Geometry check sheet. Reference: the model listing, model coordinates, mm. Face numbers are marked on the shaded views. A direction names the side the tool comes from. Round coordinates to 2 decimals unless told otherwise and drop trailing zeros. Write each loop counter-clockwise with the first axis right and the second up, starting at its lowest first coordinate (ties: lowest second). Pieces come first, ordered by that corner, then holes. Notation, with made-up numbers: M 48.5,72.5 L 74.5,72.5 A16 cw 74.5,101.5 Z; hole C 28,62 d6. An arc over 180 degrees is marked long. One line per item, written item: value. Start each with the question number.
1. Section check B-B (y = 34.5). Record the boundary of the cut face in (x, z).
2. Section check A-A (y = 82.5). Record the boundary of the cut face in (x, z), and give its area (3 significant figures).
3. Scan lines: probe 1 along X at (y, z) = (14.5, -3.25); probe 2 along X at (y, z) = (-78, 1); probe 3 along Y at (x, z) = (-19, -2.75). Record each from-to range of solid material in increasing order. Write a range as [from, to].
4. Release check for a two-part mould opening along Y. For the marked faces 5, 6 and 7 record: pulls with the +Y half, pulls with the -Y half, needs draft (parallel to the pull), parting line crosses it, or undercut.
5. Access from +Z, -Z, +X, -X, +Y, -Y to the whole of each face (thin tool, end or side, straight path). Record for the marked faces 1, 2, 3 and 4.
6. Depth check by flat-ended pin: P1, Ø6, axis at y = -48.5, z = -2, coming from the +X side; P2, Ø5, axis at y = -47.5, z = -4, coming from the -X side; P3, Ø5, axis at y = 56.5, z = 0.5, coming from the -X side. Enter the tip coordinate at first touch or a pass-through.
from build123d import *

# Parameters (mm, degrees)
SKETCH_1_W          = 49.8
SKETCH_1_H          = 190
EXTRUDE_1_DEPTH     = 5
CUT_EXTRUDE_1_DEPTH = 99.71681721
FILLET_1_R          = 5
CUT_EXTRUDE_2_DEPTH = 99.71681721
CHAMFER_2_SIZE      = 20
CUT_EXTRUDE_6_REACH = 100.717
SKETCH_7_R          = 2.1
SKETCH_3_W          = 30.2
SKETCH_3_H          = 6.2
CUT_EXTRUDE_7_DEPTH = 49
CHAMFER_3_SIZE      = 5
SKETCH_9_R          = 3.7
CUT_EXTRUDE_8_DEPTH = 5


with BuildPart() as part:
    # 草图1 → 凸台-拉伸1 (new, symmetric)
    with BuildSketch(Plane.XY):
        Rectangle(SKETCH_1_W, SKETCH_1_H)
    extrude(amount=EXTRUDE_1_DEPTH, both=True)

    # 草图4 → 切除-拉伸1 (cut, through all)
    with BuildSketch(Plane(origin=(0, 0, -5), x_dir=(-1, 0, 0), z_dir=(0, 0, -1))):
        Polygon((-24.9, 62.5), (-15, 45.352697005), (-15, -45.352697005), (-24.9, -62.5), align=None)
        Polygon((24.9, -62.5), (24.9, 62.5), (15, 45.352697005), (15, -45.352697005), align=None)
    extrude(amount=-CUT_EXTRUDE_1_DEPTH, mode=Mode.SUBTRACT)

    # 圆角1
    fillet_1_edges = [part.edges().sort_by_distance(p)[0] for p in [
        (24.9, -62.5, 0),
        (24.9, 62.5, 0),
        (15, 45.352697005, 0),
        (15, -45.352697005, 0),
        (-24.9, -62.5, 0),
        (-15, -45.352697005, 0),
        (-15, 45.352697005, 0),
        (-24.9, 62.5, 0),
        (24.9, -95, 0),
        (-24.9, -95, 0),
        (-24.9, 95, 0),
        (24.9, 95, 0),
    ]]
    fillet(fillet_1_edges, radius=FILLET_1_R)

    # 草图5 → 切除-拉伸2 (cut, through all)
    with BuildSketch(Plane(origin=(0, 0, -5), x_dir=(-1, 0, 0), z_dir=(0, 0, -1))):
        Polygon((-19.9, 90), (-19.9, 63.839745962), (-10, 46.692442967), (-10, 2.5), (-5, 2.5), (-5, 90), align=None)
        Polygon((5, 90), (19.9, 90), (19.9, 63.839745962), (10, 46.692442967), (10, 2.5), (5, 2.5), align=None)
        Polygon((19.9, -90), (19.9, -63.839745962), (10, -46.692442967), (10, -2.5), (5, -2.5), (5, -90), align=None)
        Polygon((-5, -90), (-19.9, -90), (-19.9, -63.839745962), (-10, -46.692442967), (-10, -2.5), (-5, -2.5), align=None)
    extrude(amount=-CUT_EXTRUDE_2_DEPTH, mode=Mode.SUBTRACT)

    # 倒角2
    # the kernel refuses this chamfer: 20 mm, written as the material it adds along each edge
    with BuildSketch(Plane(origin=(-19.9, 90, -5), x_dir=(-0.027495876610586147, -0.9996219169112968, 0), z_dir=(0, 0, 1))) as chamfer_2_piece_1:
        Polygon((CHAMFER_2_SIZE * 0.999621916911, CHAMFER_2_SIZE * 0.0274958766106), (-CHAMFER_2_SIZE * 0.0274958766106, CHAMFER_2_SIZE * 0.999621916911), (0, 0), align=None)
    extrude(amount=10)
    with BuildSketch(Plane(origin=(19.9, 90, -5), x_dir=(0.027495876610586147, -0.9996219169112968, 0), z_dir=(0, 0, 1))) as chamfer_2_piece_2:
        Polygon((CHAMFER_2_SIZE * 0.999621916911, -CHAMFER_2_SIZE * 0.0274958766106), (-CHAMFER_2_SIZE * 0.0274958766106, -CHAMFER_2_SIZE * 0.999621916911), (0, 0), align=None)
    extrude(amount=10)

    # 草图7 → 切除-拉伸6 (cut, up to next)
    with BuildSketch(Plane(origin=(0, 0, -5), x_dir=(-1, 0, 0), z_dir=(0, 0, -1)), mode=Mode.PRIVATE) as cut_extrude_6_sk1:
        with Locations((-20, 82.5)):
            Circle(SKETCH_7_R)
    cut_extrude_6_tool1 = extrude(cut_extrude_6_sk1.sketch, amount=-CUT_EXTRUDE_6_REACH, mode=Mode.PRIVATE) & part.part
    # 草图7 → 切除-拉伸6 (cut, up to next)
    with BuildSketch(Plane(origin=(0, 0, -5), x_dir=(-1, 0, 0), z_dir=(0, 0, -1)), mode=Mode.PRIVATE) as cut_extrude_6_sk2:
        with Locations(Location((20, 82.5, 0), (0, 0, 180))):
            Circle(SKETCH_7_R)
    cut_extrude_6_tool2 = extrude(cut_extrude_6_sk2.sketch, amount=-CUT_EXTRUDE_6_REACH, mode=Mode.PRIVATE) & part.part
    add(cut_extrude_6_tool1.solids().sort_by_distance((20, 82.5, -5))[0], mode=Mode.SUBTRACT)
    add(cut_extrude_6_tool2.solids().sort_by_distance((-20, 82.5, -5))[0], mode=Mode.SUBTRACT)

    # 草图3 → 切除-拉伸7 (cut)
    with BuildSketch(Plane.XZ.offset(95)):
        Rectangle(SKETCH_3_W, SKETCH_3_H)
    extrude(amount=-CUT_EXTRUDE_7_DEPTH, mode=Mode.SUBTRACT)

    # 倒角3
    chamfer_3_edges = [part.edges().sort_by_distance(p)[0] for p in [
        (-15.1, -46, 0),
        (15.1, -46, 0),
    ]]
    chamfer(chamfer_3_edges, length=CHAMFER_3_SIZE)

    # 草图9 → 切除-拉伸8 (cut)
    with BuildSketch(Plane(origin=(0, 0, -5), x_dir=(-1, 0, 0), z_dir=(0, 0, -1))):
        with Locations((-20, 82.5)):
            Circle(SKETCH_9_R)
        with Locations((20, 82.5)):
            Circle(SKETCH_9_R)
    extrude(amount=-CUT_EXTRUDE_8_DEPTH, mode=Mode.SUBTRACT)


solid = part.part
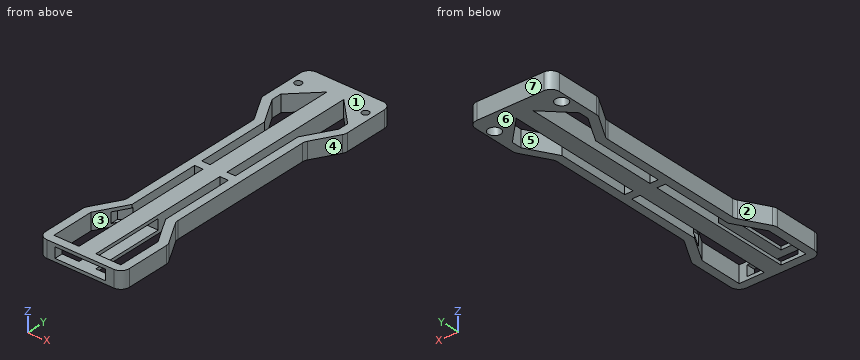
Result sheet:
1. outline: M -15,-5 L -10,-5 L -10,5 L -15,5 Z; M -5,-5 L 5,-5 L 5,5 L -5,5 Z; M 10,-5 L 15,-5 L 15,5 L 10,5 Z
2. outline: M -24.9,-5 L -23.7,-5 L -23.7,0 L -22.1,0 L -22.1,5 L -24.9,5 Z; M -17.9,0 L -16.3,0 L -16.3,-5 L -7.4,-5 L -7.4,5 L -17.9,5 Z; M -5,-5 L 5,-5 L 5,5 L -5,5 Z; M 7.4,-5 L 16.3,-5 L 16.3,0 L 17.9,0 L 17.9,5 L 7.4,5 Z; M 22.1,0 L 23.7,0 L 23.7,-5 L 24.9,-5 L 24.9,5 L 22.1,5 Z
2. area: 334 mm2
3. probe 1: x = [-15, -10], [-5, 5], [10, 15]
3. probe 2: x = [-24.9, -19.9], [19.9, 24.9]
3. probe 3: y = [-95, -90], [-62.28, -52.28], [52.28, 62.28], [70.9, 78.94], [86.06, 95]
4. face 5: undercut
4. face 6: needs draft
4. face 7: pulls with the +Y half
5. face 1: +Z, +X, -X, +Y, -Y
5. face 2: +Z, -Z, -X
5. face 3: +Z, -Z
5. face 4: +Z, -Z, +X
6. P1: stops at x = 18.55
6. P2: stops at x = -17.68
6. P3: stops at x = -22.88
